CAD build for the part. Positions are in the model's coordinates, mm. Face numbers are marked on the shaded views. A direction names the side the tool comes from. Coordinates: 2 decimals unless noted, no trailing zeros. Order: outer loops, then holes, each group sorted by start corner. A loop starts at its lowest first (then second) coordinate and runs counter-clockwise, first axis right, second up. Notation, with made-up numbers: (36, 62.25) - (43, 62.25) arc R12 ccw to (43, 75.25) - close; hole circle Ø3 at (-19, 37.5). An arc over 180 degrees is marked (long way). Use one line per item in the form item = value.
```python
from build123d import *

# Parameters (mm, degrees)
F1_DEPTH = 39
F2_R     = 2.5
F3_DEPTH = 2.748386896
F4_W     = 10
F4_H     = 10
F5_DEPTH = 3
F6_W     = 71.9977971367
F6_H     = 27.748386896
F7_DEPTH = 2.5
F8_W     = 10
F8_H     = 10
F9_DEPTH = 2.5


with BuildPart() as f1:
    # F0 (on Front) → F1 (new body, symmetric)
    with BuildSketch(Plane.XZ):
        Polygon((33.0240737289, -6.6249261405), (-2.9748248395, -6.6249261405), (-2.9748248395, -9.6249261405), (36.0251751605, -9.6249261405), (36.0251751605, 18.3750738595), (48.0240737289, 18.3750738595), (48.0240737289, 21.1234607555), (33.0240737289, 21.1234607555), align=None)
        Polygon((-2.9748248395, -9.6249261405), (-2.9748248395, -6.6249261405), (-38.9737234078, -6.6249261405), (-38.9737234078, 21.1234607555), (-53.9737234078, 21.1234607555), (-53.9737234078, 18.3750738595), (-41.9748248395, 18.3750738595), (-41.9748248395, -9.6249261405), align=None)
    extrude(amount=F1_DEPTH, both=True)

    # F2 (on face) → F3 (cut, through all)
    with BuildSketch(Plane.XY.offset(21.1234607555)):
        with Locations((42.0246244447, -24)):
            Circle(F2_R)
        with Locations((42.0246244447, 24)):
            Circle(F2_R)
        with Locations((-47.9742741236, 24)):
            Circle(F2_R)
        with Locations((-47.9742741236, -24)):
            Circle(F2_R)
    extrude(amount=-F3_DEPTH, mode=Mode.SUBTRACT)

    # F4 (on face) → F5 (cut, through all)
    with BuildSketch(Plane(origin=(0, 0, -9.6249261405), x_dir=(1, 0, 0), z_dir=(0, 0, -1))):
        with Locations((-31.4737234078, 31.5)):
            Rectangle(F4_W, F4_H)
        with Locations((-17.4737234078, 31.5)):
            Rectangle(F4_W, F4_H)
        with Locations((-3.4737234078, 31.5)):
            Rectangle(F4_W, F4_H)
        with Locations((10.5262765922, 31.5)):
            Rectangle(F4_W, F4_H)
        with Locations((24.5262765922, 31.5)):
            Rectangle(F4_W, F4_H)
        with Locations((10.5262765922, 18.9653515071)):
            Rectangle(F4_W, F4_H)
        with Locations((24.5262765922, 18.9653515071)):
            Rectangle(F4_W, F4_H)
        with Locations((-31.4737234078, 18.9653515071)):
            Rectangle(F4_W, F4_H)
        with Locations((-17.4737234078, 18.9653515071)):
            Rectangle(F4_W, F4_H)
        with Locations((-3.4737234078, 18.9653515071)):
            Rectangle(F4_W, F4_H)
        with Locations((10.5262765922, 6.4307030141)):
            Rectangle(F4_W, F4_H)
        with Locations((24.5262765922, 6.4307030141)):
            Rectangle(F4_W, F4_H)
        with Locations((-31.4737234078, 6.4307030141)):
            Rectangle(F4_W, F4_H)
        with Locations((-17.4737234078, 6.4307030141)):
            Rectangle(F4_W, F4_H)
        with Locations((-3.4737234078, 6.4307030141)):
            Rectangle(F4_W, F4_H)
        with Locations((10.5262765922, -6.1039454788)):
            Rectangle(F4_W, F4_H)
        with Locations((24.5262765922, -6.1039454788)):
            Rectangle(F4_W, F4_H)
        with Locations((-31.4737234078, -6.1039454788)):
            Rectangle(F4_W, F4_H)
        with Locations((-17.4737234078, -6.1039454788)):
            Rectangle(F4_W, F4_H)
        with Locations((-3.4737234078, -6.1039454788)):
            Rectangle(F4_W, F4_H)
        with Locations((10.5262765922, -18.6385939717)):
            Rectangle(F4_W, F4_H)
        with Locations((24.5262765922, -18.6385939717)):
            Rectangle(F4_W, F4_H)
        with Locations((-31.4737234078, -18.6385939717)):
            Rectangle(F4_W, F4_H)
        with Locations((-17.4737234078, -18.6385939717)):
            Rectangle(F4_W, F4_H)
        with Locations((-3.4737234078, -18.6385939717)):
            Rectangle(F4_W, F4_H)
        with Locations((10.5262765922, -31.1732424647)):
            Rectangle(F4_W, F4_H)
        with Locations((24.5262765922, -31.1732424647)):
            Rectangle(F4_W, F4_H)
        with Locations((-31.4737234078, -31.1732424647)):
            Rectangle(F4_W, F4_H)
        with Locations((-17.4737234078, -31.1732424647)):
            Rectangle(F4_W, F4_H)
        with Locations((-3.4737234078, -31.1732424647)):
            Rectangle(F4_W, F4_H)
    extrude(amount=-F5_DEPTH, mode=Mode.SUBTRACT)

    # F6 (on face) → F7 (join)
    with BuildSketch(Plane.XZ.offset(39)):
        with Locations((-2.9748248395, 7.2492673075)):
            Rectangle(F6_W, F6_H)
    extrude(amount=-F7_DEPTH)

    # F8 (on face) → F9 (cut, through all)
    with BuildSketch(Plane.XZ.offset(39)):
        with Locations((-26.9759262711, 14.1834607555)):
            Rectangle(F8_W, F8_H)
        with Locations((-10.9759262711, 14.1834607555)):
            Rectangle(F8_W, F8_H)
        with Locations((5.0240737289, 14.1834607555)):
            Rectangle(F8_W, F8_H)
        with Locations((21.0240737289, 14.1834607555)):
            Rectangle(F8_W, F8_H)
        with Locations((21.0240737289, 0.3084607555)):
            Rectangle(F8_W, F8_H)
        with Locations((-26.9759262711, 0.3084607555)):
            Rectangle(F8_W, F8_H)
        with Locations((-10.9759262711, 0.3084607555)):
            Rectangle(F8_W, F8_H)
        with Locations((5.0240737289, 0.3084607555)):
            Rectangle(F8_W, F8_H)
    extrude(amount=-F9_DEPTH, mode=Mode.SUBTRACT)


solid = f1.part
```
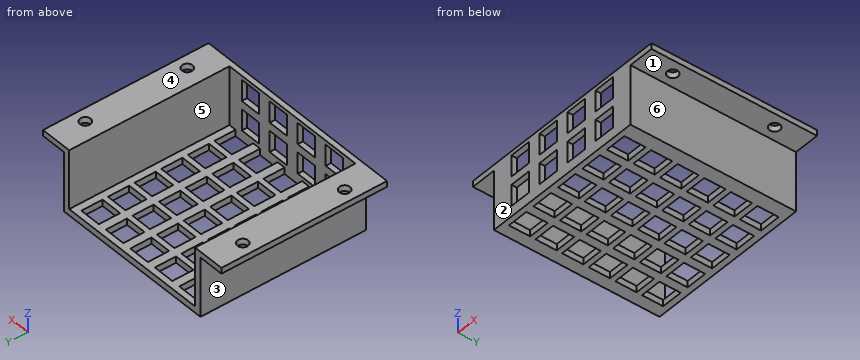
Item 1: Drill centre lines: line 1 (X direction, y = -12, z = 8.5); line 2 (Y direction, x = -4.5, z = -6); line 3 (X direction, y = -10, z = 18.5). Where is each one in solid material? Low to high. Write a range as [from, to].
Derived:
line_1 = [-41.97, -38.97], [33.02, 36.03]
line_2 = [-39, -36.5]
line_3 = [-53.97, -38.97], [33.02, 48.02]
Item 2: Drop flat-ended pins along their axis: pin 1 (3.5 mm diameter, centred on y = -5, z = -8, fed in from +X); pin 2 (1.5 mm diameter, centred on x = 5.5, y = -28, fed in from +Z); pin 3 (3 mm diameter, centred on x = -34.5, z = -3.5, fed in from +Y). Give the stop position or say it passes through.
Derived:
pin_1 = 36.03
pin_2 = -6.62
pin_3 = -36.5
Item 3: 3-axis set-ups, long thin cutter, end or side, ignore diameter. For the marked faces 1 and 2: which of +Z, -Z, +X, -X, +Y, -Y reach the whole face in a straight line?
Derived:
face_1 = -Z, +X, +Y, -Y
face_2 = +Z, -Z, +X, -X, -Y
Item 4: Cut at B-B, the plane z = -3. Write the cut outline in (x, y), plus the area to 3 significant figures.
Derived:
outline = (-41.97, -39) - (-31.98, -39) - (-31.98, -36.5) - (-38.97, -36.5) - (-38.97, 39) - (-41.97, 39) - close; (-21.98, -39) - (-15.98, -39) - (-15.98, -36.5) - (-21.98, -36.5) - close; (-5.98, -39) - (0.02, -39) - (0.02, -36.5) - (-5.98, -36.5) - close; (10.02, -39) - (16.02, -39) - (16.02, -36.5) - (10.02, -36.5) - close; (26.02, -39) - (36.03, -39) - (36.03, 39) - (33.02, 39) - (33.02, -36.5) - (26.02, -36.5) - close
area = 548 mm²
Item 5: Cut at A-A, the plane x = 12.5. Write the cut outline in (y, z).
Derived:
outline = (-39, -9.62) - (-36.5, -9.62) - (-36.5, 21.12) - (-39, 21.12) - close; (-26.5, -9.62) - (-23.97, -9.62) - (-23.97, -6.62) - (-26.5, -6.62) - close; (-13.97, -9.62) - (-11.43, -9.62) - (-11.43, -6.62) - (-13.97, -6.62) - close; (-1.43, -9.62) - (1.1, -9.62) - (1.1, -6.62) - (-1.43, -6.62) - close; (11.1, -9.62) - (13.64, -9.62) - (13.64, -6.62) - (11.1, -6.62) - close; (23.64, -9.62) - (26.17, -9.62) - (26.17, -6.62) - (23.64, -6.62) - close; (36.17, -9.62) - (39, -9.62) - (39, -6.62) - (36.17, -6.62) - close
Item 6: Two-plate mould, pull along X, no slides. Class the marked faces 3, 4, 5 and 6: +X half, -X half, draft (parallel to the pull), parting line (faces both ways), or undercut.
Derived:
face_3 = -X half
face_4 = draft
face_5 = undercut
face_6 = +X half
Item 7: Cut at C-C, the plane y = -16. State how many separate pieces and enclosed holes the cut face has, plus the area to 3 significant figures.
Derived:
separate_pieces = 6
enclosed_holes = 0
area = 317 mm²
